Work out the finished part from the listing and answer in its coordinate system (mm). Face numbers are marked on the shaded views. A direction names the side the tool comes from. Give positions to 0.01 mm unless a question says otherwise; leave off trailing zeros. Loops run counter-clockwise (first coordinate to the right, second up) from the corner with the lowest first, then second, coordinate; pieces in that order, holes last. Notation, with made-up numbers: M 78.25,78.5 L 104.25,78.5 A16 cw 104.25,91.5 Z; hole C 38.25,10.25 d9. An arc over 180 degrees is marked long. Use a Markdown table: item, result.
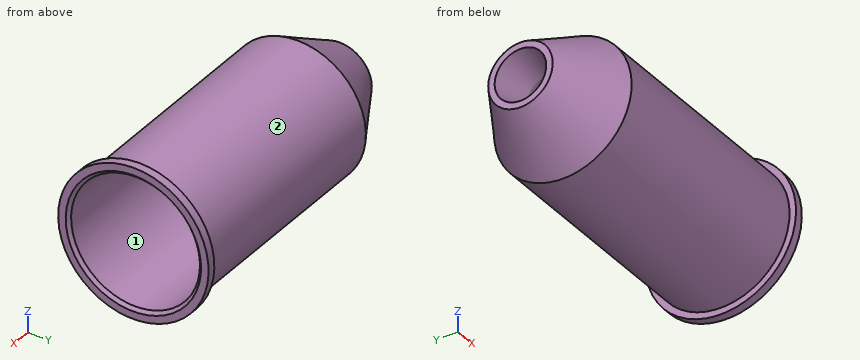
```python
from build123d import *


with BuildPart() as part:
    # Эскиз1 → Повернуть1 (revolve)
    with BuildSketch(Plane.XY, mode=Mode.PRIVATE) as revolve_1_sk:
        with BuildLine():
            Line((0, 15), (29.444863729, 32))
            Line((29.444863729, 32), (139, 32))
            Line((139, 32), (139, 35))
            Line((139, 35), (143, 35))
            Line((143, 35), (143, 31.5))
            Line((143, 31.5), (141.5, 30))
            Line((141.5, 30), (41.5, 30))
            Line((41.5, 30), (19.394228634, 7.894228634))
            ThreePointArc((19.394228634, 7.894228634), (18.573684899, 7.398584574), (17.616752191, 7.341708844))
            Line((17.616752191, 7.341708844), (16.948603844, 7.4651183))
            ThreePointArc((16.948603844, 7.4651183), (16.871071065, 7.481031521), (16.794228634, 7.5))
            Line((16.794228634, 7.5), (0, 12))
            Line((0, 12), (0, 15))
        make_face()
    revolve(revolve_1_sk.sketch.rotate(Axis((0, 0, 0), (1, 0, 0)), 90), axis=Axis((0, 0, 0), (1, 0, 0)))


solid = part.part
```
(1) Given P1, Ø3, axis at x = 95, y = -6.5, coming from the +Z side; P2, Ø12, axis at y = -22, z = -4, coming from the +X side; P3, Ø1.5, axis at x = 23, z = 16, coming from the +Y side, each flat-ended and moving along its own axis, determine where each tip first touches the part or whether it passes through.
Entries:
| item | result |
|---|---|
| P1 | stops at z = 31.61 |
| P2 | stops at x = 39.86 |
| P3 | stops at y = 24.04 |
(2) A cutting plane is placed at C-C (x = 38). Write down the section's boundary in (y, z).
Entries:
| item | result |
|---|---|
| outline | C 0,0 d64; hole C 0,0 d53 |
(3) Which of the six approach directions +Z, -Z, +X, -X, +Y, -Y give full straight-line access (tool end or side, diameter ignored) to the marked faces 1 and 2?
Entries:
| item | result |
|---|---|
| face 1 | +X |
| face 2 | -X |
(4) A cutting plane is placed at A-A (y = 0). Write down the section's boundary in (x, z).
Entries:
| item | result |
|---|---|
| outline | M 0,-15 L 29.44,-32 L 139,-32 L 139,-35 L 143,-35 L 143,-31.5 L 141.5,-30 L 41.5,-30 L 19.39,-7.89 A2 ccw 17.62,-7.34 L 16.95,-7.47 A2 ccw 16.79,-7.5 L 0,-12 Z; M 0,12 L 16.79,7.5 A2 ccw 16.95,7.47 L 17.62,7.34 A2 ccw 19.39,7.89 L 41.5,30 L 141.5,30 L 143,31.5 L 143,35 L 139,35 L 139,32 L 29.44,32 L 0,15 Z |
(5) A cutting plane is placed at D-D (x = 117.5). Write down the section's boundary in (y, z), and give its area (3 significant figures).
Entries:
| item | result |
|---|---|
| outline | C 0,0 d64; hole C 0,0 d60 |
| area | 390 mm² |
(6) Consider probe 1 along Y at (x, z) = (93.5, 0); probe 2 along Z at (x, y) = (127.5, 1); probe 3 along Y at (x, z) = (42, 11). Determine where each line is inside the solid, lowest interval first. Write a range as [from, to].
Entries:
| item | result |
|---|---|
| probe 1 | y = [-32, -30], [30, 32] |
| probe 2 | z = [-31.98, -29.98], [29.98, 31.98] |
| probe 3 | y = [-30.05, -27.91], [27.91, 30.05] |
